```python
from build123d import *

# Parameters (mm, degrees)
F1_DEPTH = 16.25
F2_R     = 1.6
F3_REACH = 20.5813230926


with BuildPart() as f1:
    # F0 (on Right) → F1 (new body, symmetric)
    with BuildSketch(Plane.YZ):
        Polygon((-10, 0), (0, 0), (0, 15), (-11, 15), align=None)
    extrude(amount=F1_DEPTH, both=True)

    f3_end = Plane(origin=(0, 0, 7.5), x_dir=(0, 0, 1), z_dir=(0, 1, 0))
    # F2 (on face) → F3 (join, up to a plane its end follows)
    with BuildSketch(Plane(origin=(0, -9.9557522124, -0.6637168142), x_dir=(1, 0, 0), z_dir=(0, -0.9977851579, -0.0665190105))):
        with BuildLine():
            Line((-18.5, 4.4318382944), (-16.25, 4.4318382944))
            Line((-16.25, 4.4318382944), (-16.25, 11.9318382944))
            Line((-16.25, 11.9318382944), (-18.5, 11.9318382944))
            ThreePointArc((-18.5, 11.9318382944), (-22.25, 8.1818382944), (-18.5, 4.4318382944))
        make_face()
        with Locations((-18.5, 8.1818382944)):
            Circle(F2_R, mode=Mode.SUBTRACT)
        with BuildLine():
            Line((16.25, 4.4318382944), (18.5, 4.4318382944))
            ThreePointArc((18.5, 4.4318382944), (22.25, 8.1818382944), (18.5, 11.9318382944))
            Line((18.5, 11.9318382944), (16.25, 11.9318382944))
            Line((16.25, 11.9318382944), (16.25, 4.4318382944))
        make_face()
        with Locations((18.5, 8.1818382944)):
            Circle(F2_R, mode=Mode.SUBTRACT)
    f3_long = extrude(amount=-F3_REACH, mode=Mode.PRIVATE)
    add(split(f3_long, bisect_by=f3_end, keep=Keep.BOTTOM, mode=Mode.PRIVATE))


solid = f1.part
```
The listing builds one solid part. Answer for the finished solid, in the listing's coordinates (mm). A direction names the side the tool comes from. Give positions to 0.01 mm unless a question says otherwise; leave off trailing zeros. Loops run counter-clockwise (first coordinate to the right, second up) from the corner with the lowest first, then second, coordinate; pieces in that order, holes last. Notation, with made-up numbers: (-23.5, 77.25) - (2.5, 77.25) arc R18 cw to (2.5, 102.25) - close; hole circle Ø9 at (-4, 81). An arc over 180 degrees is marked (long way). Answer as CSV lines item,"result". Start each with the question number.
Item 1: Each of these flat-tipped pins is pushed along its axis until it touches: pin 1 (6 mm diameter, centred on x = 5.5, z = 2, fed in from -Y); pin 2 (1 mm diameter, centred on y = -8, z = 11.5, fed in from -X); pin 3 (3.5 mm diameter, centred on y = -7.5, z = 1, fed in from +X). Where does it stop, or does it pass through?
Item 2: A cutting plane is placed at A-A on x = -8. Determine the outline of the cut face in (y, z).
Item 3: The mould has two halves that part along Z. Classify faces 1 (the face through (-17.391, -5.197, 4.095)), 2 (the face through (16.25, -6, 13)), 3 (the face through (17.32, -5.33, 8.93)): +Z half, -Z half, draft (parallel to the pull), parting line (faces both ways), or undercut.
Item 4: For faces 4 (the face through (-17.4, -5.4, 11.6)), 5 (the face through (17.4, -5.4, 11.6)), 6 (the face through (17.359, -5.197, 4.095)), 7 (the face through (0, -5, 15)), determine the directions among +Z, -Z, +X, -X, +Y, -Y from which every point of the face is accessible in a straight line to the end or side of a thin tool.
Item 5: A cutting plane is placed at C-C on z = 13.75. Determine the outline of the cut face in (x, y), then the cut area to 3 significant figures.
Item 6: Find the intervals of material crossed by line 1 (X direction, y = -9.5, z = 6.5); line 2 (X direction, y = -0.5, z = 14.75); line 3 (Z direction, x = -18, y = -5.5) (3 decimals), in increasing order. Write a range as from..to.
Item 7: A cutting plane is placed at B-B on z = 9. Count the separate pieces of the cut face and the enclosed holes in it, then the cut area to 3 significant figures.
Found:
1,pin 1,"stops at y = -10.33"
1,pin 2,"stops at x = -20.23"
1,pin 3,"stops at x = 16.25"
2,outline,"(-11, 15) - (-10, 0) - (0, 0) - (0, 15) - close"
3,face 1,"-Z half"
3,face 2,"draft"
3,face 3,"undercut"
4,face 4,"+Z, -X, -Y"
4,face 5,"+Z, +X, -Y"
4,face 6,"-Z, +X, +Y"
4,face 7,"+Z, +X, -X, +Y, -Y"
5,outline,"(-16.25, -10.92) - (16.25, -10.92) - (16.25, 0) - (-16.25, 0) - close"
5,area,"355 mm^2"
6,line 1,"x = -22.1..-19.69, -17.31..17.31, 19.69..22.1"
6,line 2,"x = -16.25..16.25"
6,line 3,"z = 4.075..6.31, 9.357..11.592"
7,separate pieces,"3"
7,enclosed holes,"0"
7,area,"422 mm^2"
